```python
from build123d import *

# Parameters (mm, degrees)
F0_R     = 5.5
F1_DEPTH = 16
F2_W     = 24
F2_H     = 4
F2_W_2   = 14
F3_DEPTH = 82.001


with BuildPart() as f1:
    # F0 (on Top) → F1 (new body)
    with BuildSketch(Plane.XY):
        with BuildLine():
            Line((-122, 0), (-14, 0))
            ThreePointArc((-14, 0), (-4.100505, 4.100505), (0, 14))
            Line((0, 14), (0, 68))
            ThreePointArc((0, 68), (-4.100505, 77.899495), (-14, 82))
            Line((-14, 82), (-122, 82))
            ThreePointArc((-122, 82), (-131.899495, 77.899495), (-136, 68))
            Line((-136, 68), (-136, 14))
            ThreePointArc((-136, 14), (-131.899495, 4.100505), (-122, 0))
        make_face()
        with Locations((-122, 14)):
            Circle(F0_R, mode=Mode.SUBTRACT)
        with Locations((-14, 14)):
            Circle(F0_R, mode=Mode.SUBTRACT)
        with Locations((-122, 68)):
            Circle(F0_R, mode=Mode.SUBTRACT)
        with Locations((-14, 68)):
            Circle(F0_R, mode=Mode.SUBTRACT)
    extrude(amount=-F1_DEPTH)

    # F2 (on face) → F3 (cut, through all)
    with BuildSketch(Plane.XZ):
        with Locations((-110, -14)):
            Rectangle(F2_W, F2_H)
        with Locations((-129, -14)):
            Rectangle(F2_W_2, F2_H)
        with Locations((-26, -14)):
            Rectangle(F2_W, F2_H)
        with Locations((-7, -14)):
            Rectangle(F2_W_2, F2_H)
        with BuildLine():
            Line((-44, -1), (-44, 0))
            Line((-44, 0), (-92, 0))
            Line((-92, 0), (-92, -1))
            ThreePointArc((-92, -1), (-91.12132, -3.12132), (-89, -4))
            Line((-89, -4), (-47, -4))
            ThreePointArc((-47, -4), (-44.87868, -3.12132), (-44, -1))
        make_face()
    extrude(amount=-F3_DEPTH, mode=Mode.SUBTRACT)


solid = f1.part
```
The listing builds one solid part. Answer for the finished solid, in the listing's coordinates (mm). A direction names the side the tool comes from. Coordinates: 2 decimals unless noted, no trailing zeros. Loops run counter-clockwise (first coordinate to the right, second up) from the corner with the lowest first, then second, coordinate; pieces in that order, holes last. Notation, with made-up numbers: M 58.25,76 L 77.25,76 A22 cw 77.25,98 Z; hole C 3,-39.75 d4. An arc over 180 degrees is marked long. Answer as CSV lines item,"result". Start each with the question number.
(1) For faces 5 (the flat face through (-19, 40, -12)), 6 (the flat face through (-69, 0, -8)), 7 (the cylindrical face through (-44.9, 40.43, -3.14)), determine the directions among +Z, -Z, +X, -X, +Y, -Y from which every point of the face is accessible in a straight line to the end or side of a thin tool.
(2) The part is cut by section B-B (y = 40). Give the vertices of the cut face in (x, z).
(3) The part is cut by section A-A (y = 70). Give the vertices of the cut face in (x, z), and give its area (3 significant figures).
(4) Given pin 1 (11.5 mm diameter, centred on x = -27.5, y = 33, fed in from -Z); pin 2 (3 mm diameter, centred on y = 30.5, z = -14, fed in from +X); pin 3 (4.5 mm diameter, centred on y = 36, z = -15, fed in from -X); pin 4 (6.5 mm diameter, centred on x = -122, y = 14, fed in from -Z), each flat-ended and moving along its own axis, determine where each tip first touches the part or whether it passes through.
(5) The part is cut by section C-C (x = -68.5). Give the vertices of the cut face in (y, z).
(6) The mould has two halves that part along Y. Classify faces 1 (the cylindrical face through (-131.8, 78, -5.9)), 2 (the cylindrical face through (-126.05, 71.72, -5.92)), 3 (the cylindrical face through (-4.2, 4, -5.9)), 4 (the cylindrical face through (-11.5, 9.1, -5.9)): pulls with the +Y half, pulls with the -Y half, needs draft (parallel to the pull), parting line crosses it, or undercut.
(7) Find the intervals of material crossed by L1, parallel to Y at x = -14, z = -7; L2, parallel to Y at x = -16.5, z = -2.25; L3, parallel to Z at x = -114.5, y = 30.5, in increasing order. Write a range as [from, to].
Determined:
1,face 5,"-Z, +X, +Y, -Y"
1,face 6,"+Z, -Z, +X, -X, -Y"
1,face 7,"+Z, +Y, -Y"
2,outline,"M -136,-12 L -98,-12 L -98,-16 L -38,-16 L -38,-12 L 0,-12 L 0,0 L -44,0 L -44,-1 A3 cw -47,-4 L -89,-4 A3 cw -92,-1 L -92,0 L -136,0 Z"
3,outline,"M -135.86,-12 L -127.12,-12 L -127.12,0 L -135.86,0 Z; M -116.88,-12 L -98,-12 L -98,-16 L -38,-16 L -38,-12 L -19.12,-12 L -19.12,0 L -44,0 L -44,-1 A3 cw -47,-4 L -89,-4 A3 cw -92,-1 L -92,0 L -116.88,0 Z; M -8.88,-12 L -0.14,-12 L -0.14,0 L -8.88,0 Z"
3,area,"1,430 mm2"
4,pin 1,"z = -12"
4,pin 2,"x = -38"
4,pin 3,"x = -98"
4,pin 4,"through"
5,outline,"M 0,-16 L 82,-16 L 82,-4 L 0,-4 Z"
6,face 1,"pulls with the +Y half"
6,face 2,"undercut"
6,face 3,"pulls with the -Y half"
6,face 4,"undercut"
7,L1,"[0, 8.5], [19.5, 62.5], [73.5, 82]"
7,L2,"[0, 9.1], [18.9, 63.1], [72.9, 82]"
7,L3,"[-12, 0]"
